Job drawing, mm, ordinate dimensions from the low corner. One solid piece. Round coordinates to 2 decimals unless told otherwise and drop trailing zeros. Loops run counter-clockwise (first coordinate to the right, second up) from the corner with the lowest first, then second, coordinate; pieces in that order, holes last.
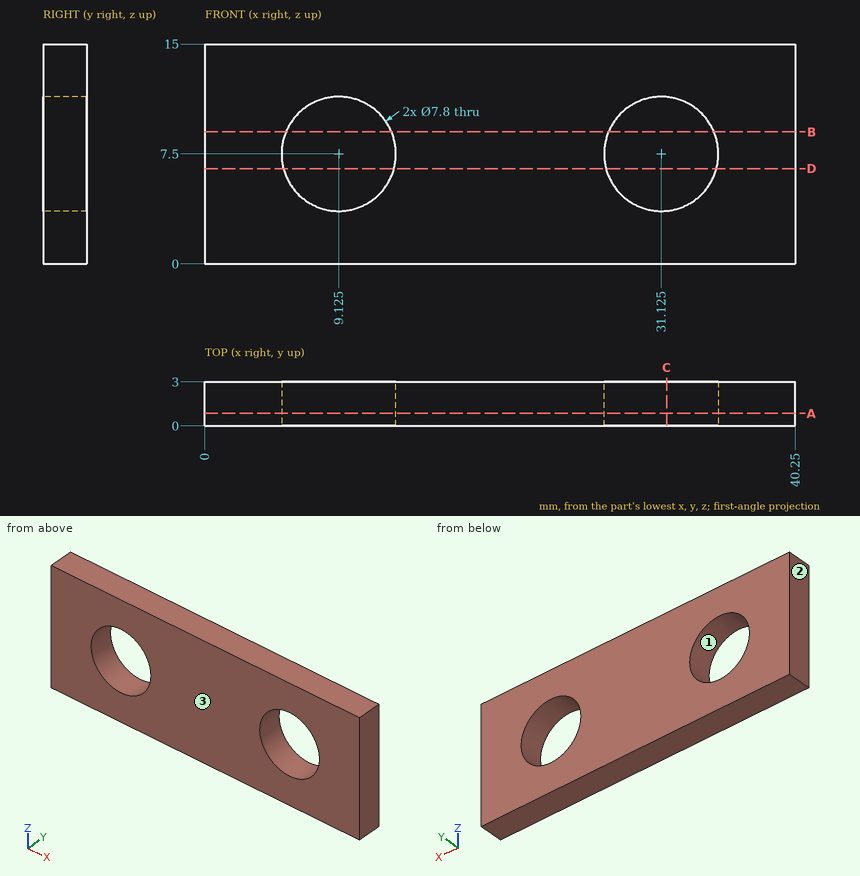
Item 1: Two-plate mould, pull along X, no slides. Class the marked faces 1, 2 and 3: released by +X, released by -X, zero draft, split by the parting line, or undercut.
Answers follow:
face 1: undercut
face 2: released by -X
face 3: zero draft
Item 2: Cut at B-B, the plane z = 9. Give the cut face in (x, y) (3 decimals).
Answers follow:
outline: (0, 0) - (5.525, 0) - (5.525, 3) - (0, 3) - close; (12.725, 0) - (27.525, 0) - (27.525, 3) - (12.725, 3) - close; (34.725, 0) - (40.25, 0) - (40.25, 3) - (34.725, 3) - close
Item 3: Cut at C-C, the plane x = 31.5. Give the cut face in (y, z).
Answers follow:
outline: (0, 0) - (3, 0) - (3, 3.62) - (0, 3.62) - close; (0, 11.38) - (3, 11.38) - (3, 15) - (0, 15) - close
Item 4: Probe line 1 (X direction, y = 2.4, z = 9.5); line 2 (X direction, y = 1.05, z = 9.75); line 3 (Z direction, x = 29, y = 1.5). List the from-to ranges inside material, lowest first.
Answers follow:
line 1: x = 0 to 5.78, 12.47 to 27.78, 34.47 to 40.25
line 2: x = 0 to 5.94, 12.31 to 27.94, 34.31 to 40.25
line 3: z = 0 to 4.23, 10.77 to 15
Item 5: Cut at A-A, the plane y = 0.85. Give the cut face in (x, z) (3 decimals).
Answers follow:
outline: (0, 0) - (40.25, 0) - (40.25, 15) - (0, 15) - close; hole circle Ø7.8 at (9.125, 7.5); hole circle Ø7.8 at (31.125, 7.5)
Item 6: Cut at D-D, the plane z = 6.5. Give the cut face in (x, y).
Answers follow:
outline: (0, 0) - (5.36, 0) - (5.36, 3) - (0, 3) - close; (12.89, 0) - (27.36, 0) - (27.36, 3) - (12.89, 3) - close; (34.89, 0) - (40.25, 0) - (40.25, 3) - (34.89, 3) - close
Item 7: Flat gauge pins, fed straight in: P1, Ø9, axis at x = 9.125, z = 7.5, coming from the -Y side; P2, Ø4.5, axis at x = 31.125, z = 7.5, coming from the -Y side. Where does each tip first touch, or does it go through?
Answers follow:
P1: stops at y = 0
P2: passes through
